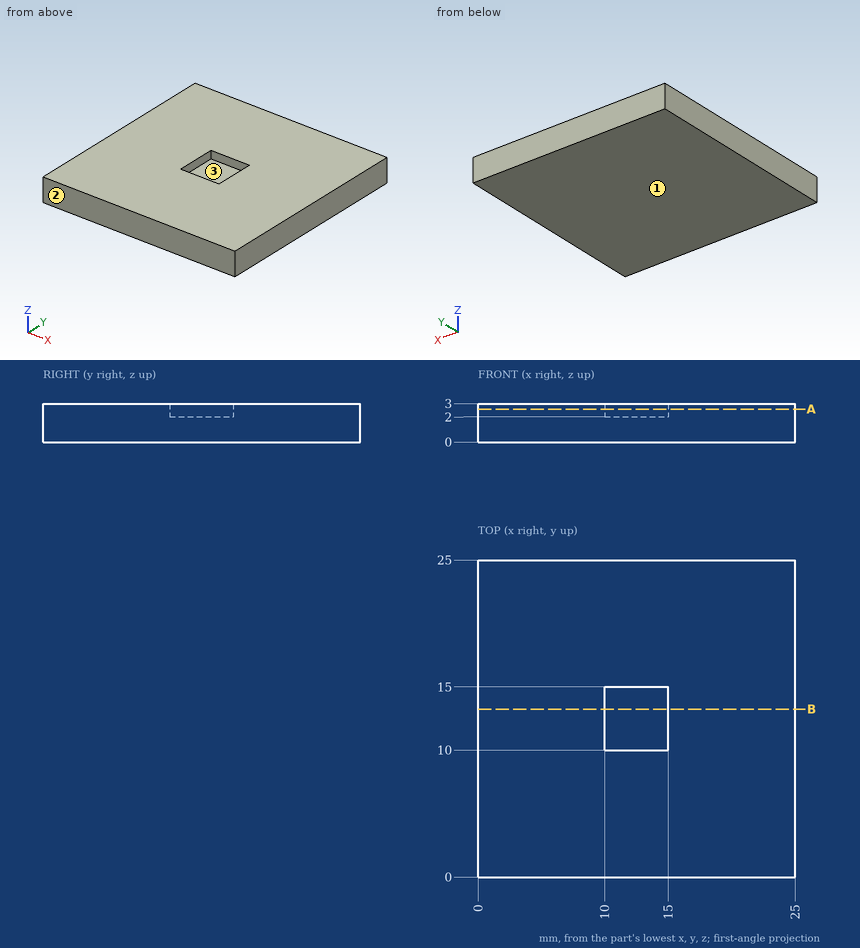
For this review, use the dimensioned drawing (mm, ordinates from the lowest corner) and the shaded views. Coordinates: 2 decimals unless noted, no trailing zeros. Loops run counter-clockwise (first coordinate to the right, second up) from the corner with the lowest first, then second, coordinate; pieces in that order, holes last. Notation, with made-up numbers: (22.25, -2) -> (42.25, -2) arc R15 ccw to (42.25, 23) -> close; hole circle Ø2 at (49, -28.75). An arc over 180 degrees is marked (long way). Use a Markdown table: item, result. Add a question column.
Item 1: We need section A-A, the plane z = 2.6. Write out the cut boundary in (x, y).
Item 2: We need section B-B, the plane y = 13.25. Write out the cut boundary in (x, z), and give its area (3 significant figures).
Item 3: Clearance check with a flat-ended pin moving along its axis: P1, Ø2.5, axis at x = 13.5, y = 12, coming from the +Z side. State where the tip first meets the part, or that it passes through.
Item 4: Wall thickness on L1, parallel to Y at x = 13, z = 2.75: over which ranges is the line inside the solid? List them lowest first. Write a range as from..to.
Item 5: The part is to be moulded in two halves that separate along Y. For the marked faces 1, 2 and 3, say which applies: +Y half, -Y half, draft (parallel to the pull), parting line (faces both ways), or undercut.
Numbers:
| question | item | result |
|---|---|---|
| 1 | outline | (0, 0) -> (25, 0) -> (25, 25) -> (0, 25) -> close; hole (10, 10) -> (15, 10) -> (15, 15) -> (10, 15) -> close |
| 2 | outline | (0, 0) -> (25, 0) -> (25, 3) -> (15, 3) -> (15, 2) -> (10, 2) -> (10, 3) -> (0, 3) -> close |
| 2 | area | 70.0 mm^2 |
| 3 | P1 | stops at z = 2 |
| 4 | L1 | y = 0..10, 15..25 |
| 5 | face 1 | draft |
| 5 | face 2 | -Y half |
| 5 | face 3 | undercut |
